For this review, take the finished solid that the model builds, in its own axes (mm). A direction names the side the tool comes from. Coordinates: 2 decimals unless noted, no trailing zeros. Order: outer loops, then holes, each group sorted by start corner. A loop starts at its lowest first (then second) coordinate and runs counter-clockwise, first axis right, second up. Notation, with made-up numbers: (-28, 49.25) -> (-14, 49.25) arc R21 cw to (-14, 60.25) -> close; hole circle Ø1 at (-12.5, 74.25). An arc over 180 degrees is marked (long way). Return JSON: item names as keys, results as strings. Group by question number.
Item 1: Take a section at D-D (y = -3.5). Write out the cut boundary in (x, z).
Item 2: Take a section at A-A (x = 2.5). Write out the cut boundary in (y, z), then the cut area to 4 significant figures.
Item 3: For line 1 along Y through (x, z) = (2.5, -3.95); line 2 along X through (y, z) = (-3.95, 2.25); line 3 along Z through (x, y) = (4.3, -1.75), list the stretches that pass through material, from the lowest coordinate up.
Item 4: Take a section at B-B (z = 2.25). Write out the cut boundary in (x, y), then the cut area to 3 significant figures.
Item 5: Machinability: for faces 5 (the flat face through (2, -3.25, 0)), 6 (the flat face through (0, -1.7, -3.5)), which of the approach directions +Z, -Z, +X, -X, +Y, -Y give a long, thin tool a straight path to every point of the face, cutting with its end or side? Answer none if there is none.
Item 6: Draft analysis for pull direction X (two halves, no side actions). For faces 1 (the cylindrical face through (0.88, 2.76, -4.01)), 2 (the cylindrical face through (3.01, -4.01, 0.63)), 3 (the flat face through (2, -4, 4.75)), 4 (the flat face through (5, -1.7, -3.5)), state which applies: +X half, -X half, draft (parallel to the pull), parting line (faces both ways), or undercut.
Item 7: Insertion check: pin 1 (3 mm diameter, centred on x = 2, z = -1.5, fed in from +Y); pin 2 (1.5 mm diameter, centred on x = 2, y = 0.5, fed in from +Z). Each pin has a flat end and moves straight along its axis. Give the tip position at first contact, or say it passes through.
```python
from build123d import *

# Parameters (mm, degrees)
BOSS_EXTRUDE1_DEPTH = 5
SKETCH2_R           = 1.7
CUT_EXTRUDE1_DEPTH  = 12.739356882
SKETCH3_R           = 1.7
CUT_EXTRUDE2_DEPTH  = 12.739356882


with BuildPart() as part:
    # Sketch1 → Boss-Extrude1 (new body)
    with BuildSketch(Plane(origin=(0, 0, 0), x_dir=(0, 0, -1), z_dir=(1, 0, 0))):
        Polygon((-4.75, -3.25), (-4.75, -4.75), (4.75, -4.75), (4.75, 4.75), (3.25, 4.75), (3.25, -3.25), align=None)
    extrude(amount=BOSS_EXTRUDE1_DEPTH)

    # Sketch2 → Cut-Extrude1 (cut, through all)
    with BuildSketch(Plane(origin=(0, 0, -4.75), x_dir=(-1, 0, 0), z_dir=(0, 0, -1))):
        with Locations((-2.5, 2.25)):
            Circle(SKETCH2_R)
    extrude(amount=-CUT_EXTRUDE1_DEPTH, mode=Mode.SUBTRACT)

    # Sketch3 → Cut-Extrude2 (cut, through all)
    with BuildSketch(Plane.XZ.offset(4.75)):
        with Locations(Location((2.5, 2.25, 0), (0, 0, 270))):
            Circle(SKETCH3_R)
    extrude(amount=-CUT_EXTRUDE2_DEPTH, mode=Mode.SUBTRACT)


solid = part.part
```
Findings below:
{
 "1": {"outline": "(0, -4.75) -> (5, -4.75) -> (5, 4.75) -> (0, 4.75) -> close; hole circle Ø3.4 at (2.5, 2.25)"},
 "2": {"outline": "(-4.75, -4.75) -> (0.55, -4.75) -> (0.55, -3.25) -> (-3.25, -3.25) -> (-3.25, 0.55) -> (-4.75, 0.55) -> close; (-4.75, 3.95) -> (-3.25, 3.95) -> (-3.25, 4.75) -> (-4.75, 4.75) -> close; (3.95, -4.75) -> (4.75, -4.75) -> (4.75, -3.25) -> (3.95, -3.25) -> close", "area": "16.05 mm2"},
 "3": {"line 1": "y = -4.75 to 0.55, 3.95 to 4.75", "line 2": "x = 0 to 0.8, 4.2 to 5", "line 3": "z = -4.75 to -3.25"},
 "4": {"outline": "(0, -4.75) -> (0.8, -4.75) -> (0.8, -3.25) -> (0, -3.25) -> close; (4.2, -4.75) -> (5, -4.75) -> (5, -3.25) -> (4.2, -3.25) -> close", "area": "2.40 mm2"},
 "5": {"face 5": "+Z, +X, -X, +Y", "face 6": "+Z, -Z, -X, +Y, -Y"},
 "6": {"face 1": "undercut", "face 2": "undercut", "face 3": "draft", "face 4": "+X half"},
 "7": {"pin 1": "stops at y = -3.25", "pin 2": "stops at z = -3.25"}
}
